Geometry: final body of the model. Coordinates: model frame, mm. A direction names the side the tool comes from. Round coordinates to 2 decimals unless told otherwise and drop trailing zeros. Loops run counter-clockwise (first coordinate to the right, second up) from the corner with the lowest first, then second, coordinate; pieces in that order, holes last. Notation, with made-up numbers: M 81,-20 L 123,-20 A27 ccw 123,-4 Z; hole C 38.5,74.5 d6. An arc over 180 degrees is marked long. Answer as a JSON object with one key per item and string values.
from build123d import *

# Parameters (mm, degrees)
SKETCH1_W           = 65
SKETCH1_H           = 25
BOSS_EXTRUDE1_DEPTH = 25
SKETCH2_W           = 25
SKETCH2_H           = 25
BOSS_EXTRUDE2_DEPTH = 20
SKETCH3_W           = 25
SKETCH3_H           = 25
SKETCH3_W_2         = 23
SKETCH3_H_2         = 23
CUT_EXTRUDE2_DEPTH  = 20
SKETCH4_W           = 25
SKETCH4_H           = 25
SKETCH4_W_2         = 23
SKETCH4_H_2         = 23
CUT_EXTRUDE3_DEPTH  = 20
SKETCH5_W           = 25
SKETCH5_H           = 25
SKETCH5_W_2         = 23
SKETCH5_H_2         = 23
CUT_EXTRUDE4_DEPTH  = 20
SKETCH6_W           = 18
SKETCH6_H           = 18
CUT_EXTRUDE5_DEPTH  = 224.89200104
SKETCH7_W           = 18
SKETCH7_H           = 18
CUT_EXTRUDE6_DEPTH  = 41.5


with BuildPart() as part:
    # Sketch1 → Boss-Extrude1 (new body)
    with BuildSketch(Plane.XY):
        with Locations((141.619238947, -196.969874038)):
            Rectangle(SKETCH1_W, SKETCH1_H)
    extrude(amount=BOSS_EXTRUDE1_DEPTH)

    # Sketch2 → Boss-Extrude2 (add)
    with BuildSketch(Plane.XY.offset(25)):
        with Locations((141.619238947, -196.969874038)):
            Rectangle(SKETCH2_W, SKETCH2_H)
    extrude(amount=BOSS_EXTRUDE2_DEPTH)

    # Sketch3 → Cut-Extrude2 (cut)
    with BuildSketch(Plane.XY.offset(45)):
        with Locations((141.619238947, -196.969874038)):
            Rectangle(SKETCH3_W, SKETCH3_H)
        with Locations((141.619238947, -196.969874038)):
            Rectangle(SKETCH3_W_2, SKETCH3_H_2, mode=Mode.SUBTRACT)
    extrude(amount=-CUT_EXTRUDE2_DEPTH, mode=Mode.SUBTRACT)

    # Sketch4 → Cut-Extrude3 (cut)
    with BuildSketch(Plane.ZY.offset(-109.119238947)):
        with Locations((12.5, -196.969874038)):
            Rectangle(SKETCH4_W, SKETCH4_H)
        with Locations((12.5, -196.969874038)):
            Rectangle(SKETCH4_W_2, SKETCH4_H_2, mode=Mode.SUBTRACT)
    extrude(amount=-CUT_EXTRUDE3_DEPTH, mode=Mode.SUBTRACT)

    # Sketch5 → Cut-Extrude4 (cut)
    with BuildSketch(Plane(origin=(174.119238947, 0, 0), x_dir=(0, 0, -1), z_dir=(1, 0, 0))):
        with Locations((-12.5, -196.969874038)):
            Rectangle(SKETCH5_W, SKETCH5_H)
        with Locations((-12.5, -196.969874038)):
            Rectangle(SKETCH5_W_2, SKETCH5_H_2, mode=Mode.SUBTRACT)
    extrude(amount=-CUT_EXTRUDE4_DEPTH, mode=Mode.SUBTRACT)

    # Sketch6 → Cut-Extrude5 (cut, through all)
    with BuildSketch(Plane(origin=(174.119238947, 0, 0), x_dir=(0, 0, -1), z_dir=(1, 0, 0))):
        with Locations((-12.5, -196.969874038)):
            Rectangle(SKETCH6_W, SKETCH6_H)
    extrude(amount=-CUT_EXTRUDE5_DEPTH, mode=Mode.SUBTRACT)

    # Sketch7 → Cut-Extrude6 (cut)
    with BuildSketch(Plane.XY.offset(45)):
        with Locations((141.619238947, -196.969874038)):
            Rectangle(SKETCH7_W, SKETCH7_H)
    extrude(amount=-CUT_EXTRUDE6_DEPTH, mode=Mode.SUBTRACT)


solid = part.part
1) Section query B-B (z = 8). Return the cut outline in (x, y), and give its area (3 significant figures).
Results:
{"outline": "M 109.12,-208.47 L 129.12,-208.47 L 129.12,-209.47 L 154.12,-209.47 L 154.12,-208.47 L 174.12,-208.47 L 174.12,-205.97 L 109.12,-205.97 Z; M 109.12,-187.97 L 174.12,-187.97 L 174.12,-185.47 L 154.12,-185.47 L 154.12,-184.47 L 129.12,-184.47 L 129.12,-185.47 L 109.12,-185.47 Z", "area": "375 mm2"}
2) Pin query (flat end, axial travel): P1, Ø5, axis at x = 162, z = 19.5, coming from the +Y side; P2, Ø10, axis at x = 162, y = -192, coming from the +Z side; P3, Ø4, axis at x = 127, z = 38, coming from the +Y side; P4, Ø9, axis at x = 148, y = -198, coming from the +Z side. Return the tip coordinate at first contact, or that it passes through.
Results:
{"P1": "y = -185.47", "P2": "z = 24", "P3": "through", "P4": "z = 45"}
3) Reachability of faces 4 (the flat face through (132.619, -197, 33)), 5 (the flat face through (142, -197, 3.5)), 6 (the flat face through (164, -208.47, 13)), 7 (the flat face through (119, -197, 24)) from +Z, -Z, +X, -X, +Y, -Y: full face, straight path, thin tool, end or side. Return the list, or none.
Results:
{"face 4": "+Z", "face 5": "+X, -X", "face 6": "+Z, -Z, +X, -Y", "face 7": "+Z, -X, +Y, -Y"}
4) Pull-direction query (Y, two-part tool) for faces 1 (the flat face through (119, -208.47, 12)), 2 (the flat face through (164, -197, 24)), 3 (the flat face through (142, -205.97, 20)); classes: +Y half, -Y half, draft (parallel to the pull), parting line (faces both ways), or undercut.
Results:
{"face 1": "-Y half", "face 2": "draft", "face 3": "undercut"}
5) Section query C-C (x = 131.5). Return the cut outline in (y, z).
Results:
{"outline": "M -209.47,0 L -184.47,0 L -184.47,25 L -185.47,25 L -185.47,45 L -208.47,45 L -208.47,25 L -209.47,25 Z; hole M -205.97,3.5 L -187.97,3.5 L -187.97,21.5 L -205.97,21.5 Z"}
6) Ray query, line 1 (Y direction, x = 150, z = 9.5); line 2 (Z direction, x = 123, y = -196); line 3 (X direction, y = -201, z = 31). Return the intervals inside material, ascending.
Results:
{"line 1": "-209.47 to -205.97, -187.97 to -184.47", "line 2": "1 to 3.5, 21.5 to 24", "line 3": "130.12 to 132.62, 150.62 to 153.12"}
7) Section query D-D (z = 35). Return the cut outline in (x, y), and give its area (3 significant figures).
Results:
{"outline": "M 130.12,-208.47 L 153.12,-208.47 L 153.12,-185.47 L 130.12,-185.47 Z; hole M 132.62,-205.97 L 150.62,-205.97 L 150.62,-187.97 L 132.62,-187.97 Z", "area": "205 mm2"}
8) Section query A-A (y = -204.25). Return the cut outline in (x, z).
Results:
{"outline": "M 109.12,1 L 129.12,1 L 129.12,0 L 154.12,0 L 154.12,1 L 174.12,1 L 174.12,3.5 L 109.12,3.5 Z; M 109.12,21.5 L 132.62,21.5 L 132.62,45 L 130.12,45 L 130.12,25 L 129.12,25 L 129.12,24 L 109.12,24 Z; M 150.62,21.5 L 174.12,21.5 L 174.12,24 L 154.12,24 L 154.12,25 L 153.12,25 L 153.12,45 L 150.62,45 Z"}
